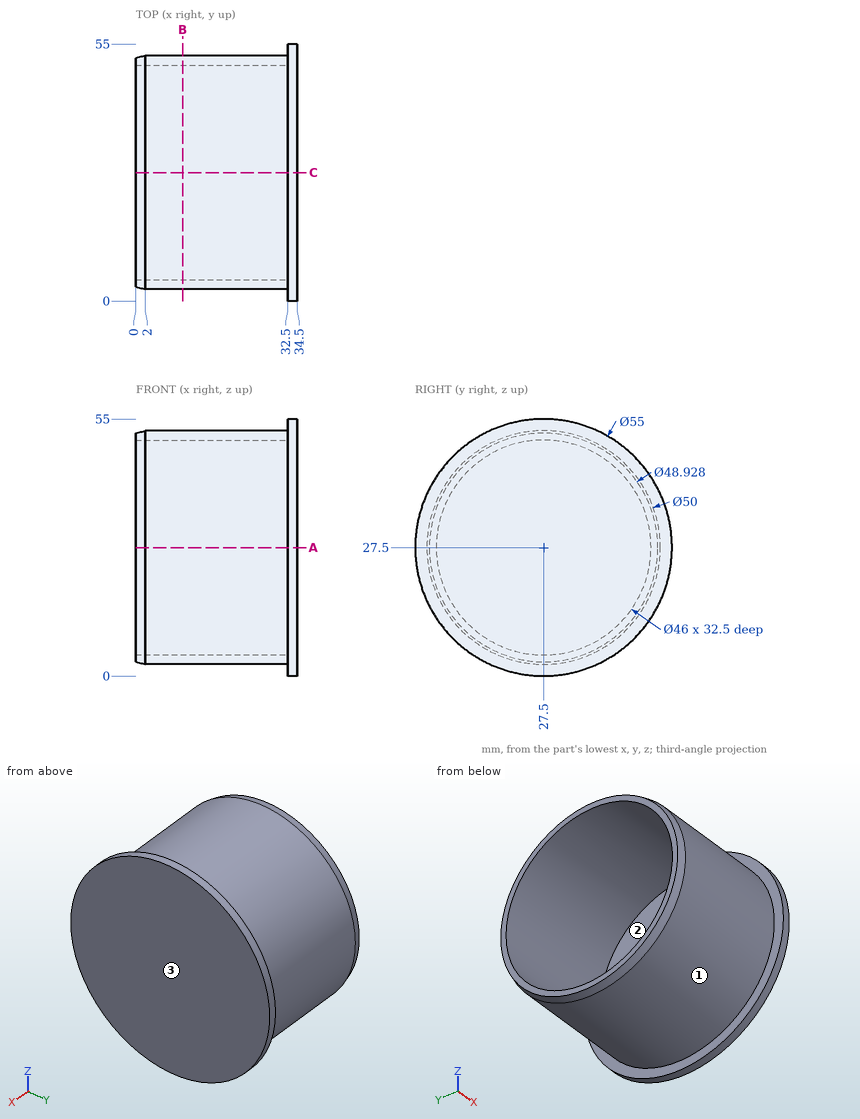
Could you check a few things on this drawing? It's one solid part, dimensions in mm from its lowest x, y, z. Give positions to 0.01 mm unless a question says otherwise; leave off trailing zeros. Write each loop counter-clockwise with the first axis right and the second up, starting at its lowest first coordinate (ties: lowest second). Pieces come first, ordered by that corner, then holes. Notation, with made-up numbers: (7.5, 48) - (57.5, 48) arc R10 cw to (57.5, 53) - close; hole circle Ø10 at (-20, 42.25). An arc over 180 degrees is marked (long way). Use CSV: the item, a comma, the result in double quotes. Start each with the question number.
Item 1: If I drill on line 1 along Y through (x, z) = (20, 27) (1 decimal); line 2 along X through (y, z) = (45.5, 34), over which ranges is the centre line in solid material (lowest first)?
Item 2: I want a section at B-B, the plane x = 10. Please give me the cut outline in (y, z).
Item 3: I want a section at A-A, the plane z = 27.5. Please give me the cut outline in (x, y), then the cut area to 3 significant figures.
Item 4: I'm going to push flat-ended pins straight in: pin 1 (8 mm diameter, centred on x = 30.5, z = 46, fed in from -Y) (1 decimal); pin 2 (1.5 mm diameter, centred on x = 13, y = 18.5, fed in from +Z); pin 3 (10 mm diameter, centred on y = 27, z = 28, fed in from -X). Where does each tip first touch, or does it pass through?
Item 5: If we mould it in two halves opening along Z, with no side actions, what happens to the marked faces 1, 2 and 3? For each: pulls with the +Z half, pulls with the -Z half, needs draft (parallel to the pull), parting line crosses it, or undercut.
Findings:
1,line 1,"y = 2.5 to 4.5, 50.5 to 52.5"
1,line 2,"x = 32.5 to 34.5"
2,outline,"circle Ø50 at (27.5, 27.5); hole circle Ø46 at (27.5, 27.5)"
3,outline,"(0, 3.04) - (2, 2.5) - (32.5, 2.5) - (32.5, 0) - (34.5, 0) - (34.5, 55) - (32.5, 55) - (32.5, 52.5) - (2, 52.5) - (0, 51.96) - (0, 50.5) - (32.5, 50.5) - (32.5, 4.5) - (0, 4.5) - close"
3,area,"239 mm2"
4,pin 1,"stops at y = 4.5"
4,pin 2,"stops at z = 51.1"
4,pin 3,"stops at x = 32.5"
5,face 1,"parting line crosses it"
5,face 2,"undercut"
5,face 3,"needs draft"
